Design review of the part shown in the three views and the two pictorial views. Dimensions are in mm from the part's minimum x, y and z. A direction names the side the tool comes from. Round coordinates to 2 decimals unless told otherwise and drop trailing zeros. Loops run counter-clockwise (first coordinate to the right, second up) from the corner with the lowest first, then second, coordinate; pieces in that order, holes last.
1) Take a section at A-A (z = 94). State the section outline as (x, y) points, then the cut area to 3 significant figures.
2) Wall thickness on L1, parallel to X at y = 63, z = 19; L2, parallel to Z at x = 38, y = 67.5; L3, parallel to Z at x = 4, y = 44: over which ranges is each line inside the solid? List them lowest first.
3) Take a section at D-D (x = 10). State the section outline as (y, z) points, then the cut area to 3 significant figures.
4) Mouldability with a two-part tool opening along X and no side actions: class the marked faces 3, 4 and 5 as pulls with the +X half, pulls with the -X half, needs draft (parallel to the pull), parting line crosses it, or undercut.
5) Take a section at C-C (x = 16.5). State the section outline as (y, z) points, then the cut area to 3 significant figures.
6) Take a section at B-B (y = 44). State the section outline as (x, z) points, then the cut area to 3 significant figures.
7) Insertion check: pin 1 (1.5 mm diameter, centred on x = 12, y = 53.5, fed in from -Z); pin 2 (6 mm diameter, centred on x = 27.5, y = 7.5, fed in from -Z). Each pin has a flat end and moves straight along its axis. Give the tip position at first contact, or say it passes through.
8) Tool access review of the marked faces 1 and 2: name each direction out of +Z, -Z, +X, -X, +Y, -Y from which nothing blocks a thin tool from reaching the whole face with its end or side.
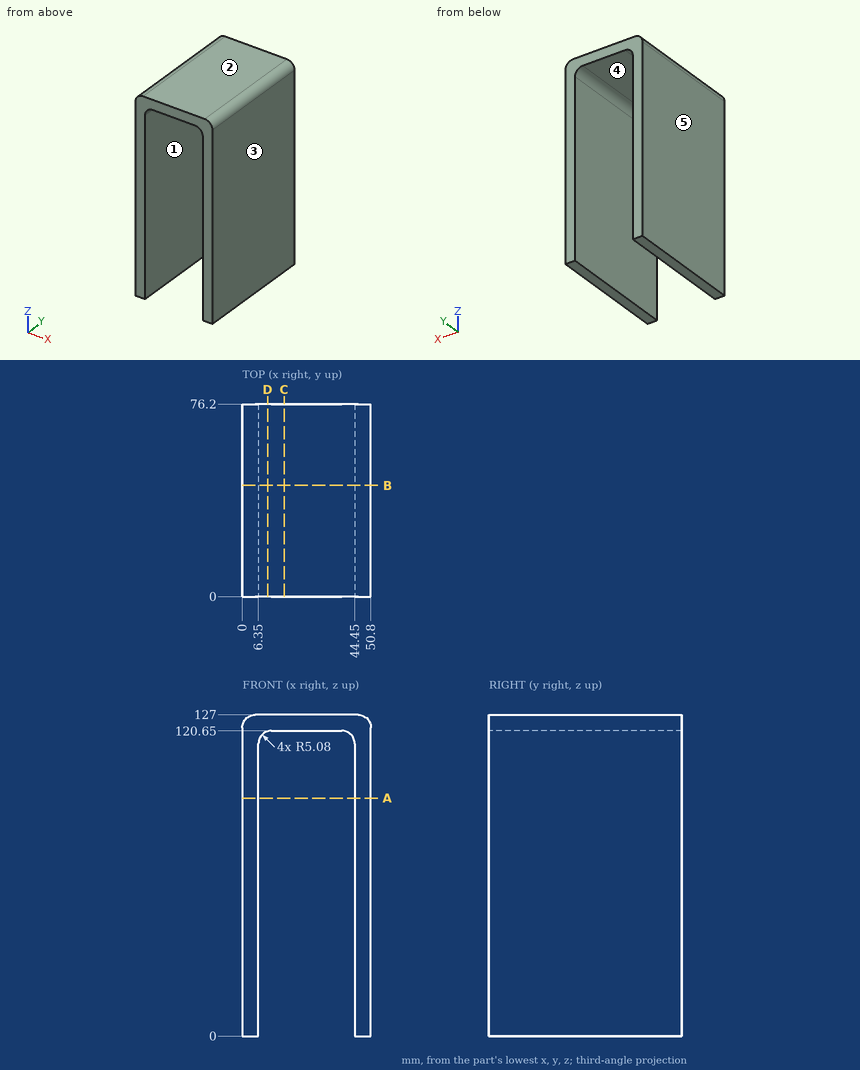
Response:
1. outline: (0, 0) - (6.35, 0) - (6.35, 76.2) - (0, 76.2) - close; (44.45, 0) - (50.8, 0) - (50.8, 76.2) - (44.45, 76.2) - close
1. area: 968 mm2
2. L1: x = 0 to 6.35, 44.45 to 50.8
2. L2: z = 120.65 to 127
2. L3: z = 0 to 126.88
3. outline: (0, 120.44) - (76.2, 120.44) - (76.2, 127) - (0, 127) - close
3. area: 500 mm2
4. face 3: pulls with the +X half
4. face 4: undercut
4. face 5: pulls with the -X half
5. outline: (0, 120.65) - (76.2, 120.65) - (76.2, 127) - (0, 127) - close
5. area: 484 mm2
6. outline: (0, 0) - (6.35, 0) - (6.35, 115.57) arc R5.08 cw to (11.43, 120.65) - (39.37, 120.65) arc R5.08 cw to (44.45, 115.57) - (44.45, 0) - (50.8, 0) - (50.8, 121.92) arc R5.08 ccw to (45.72, 127) - (5.08, 127) arc R5.08 ccw to (0, 121.92) - close
6. area: 1,850 mm2
7. pin 1: stops at z = 120.65
7. pin 2: stops at z = 120.65
8. face 1: -Z, +Y, -Y
8. face 2: +Z, +X, -X, +Y, -Y
